The model under review builds one solid part; all positions refer to its coordinate system, in mm. Face numbers are marked on the shaded views. A direction names the side the tool comes from. Coordinates: 2 decimals unless noted, no trailing zeros. Write each loop counter-clockwise with the first axis right and the second up, starting at its lowest first coordinate (ties: lowest second). Pieces come first, ordered by that corner, then holes.
1) Add section A-A, the plane y = 0. State the section outline as (x, z) points.
2) Add section C-C, the plane x = -4. State the section outline as (y, z) points, then the cut area to 3 significant figures.
3) Add section B-B, the plane z = 5.75. State the section outline as (x, y) points, then the cut area to 3 significant figures.
4) Mouldability with a two-part tool opening along Z and no side actions: class the marked faces 3, 4 and 5 as released by +Z, released by -Z, zero draft, split by the parting line, or undercut.
5) Machinability: for the marked faces 1 and 2, which of the approach directions +Z, -Z, +X, -X, +Y, -Y give a long, thin tool a straight path to every point of the face, cutting with its end or side? Answer none if there is none.
6) For P1, Ø19.5, axis at x = -12.5, y = -21.65, coming from the +Z side; P2, Ø14.5, axis at x = -12.5, y = 21.65, coming from the +Z side; P3, Ø3, axis at x = -28.5, z = 10, coming from the +Y side; P4, Ø2, axis at y = 18.5, z = 9, coming from the -X side, all flat-tipped, find the tip position at first contact; note any pin that passes through.
7) Add section D-D, the plane y = -21.65. State the section outline as (x, z) points.
8) For line 1 (X direction, y = 6, z = 5.5); line 2 (Y direction, x = 0.5, z = 4.5); line 3 (Y direction, x = -12.5, z = 1.15), list the stretches that pass through material, from the lowest coordinate up.
from build123d import *

# Parameters (mm, degrees)
SKETCH_1_R     = 37.5
PAD_1_DEPTH    = 11
SKETCH_2_R     = 15
POCKET_2_DEPTH = 11.001
SKETCH_3_R     = 4.5
POCKET_3_DEPTH = 11.001
SKETCH_4_R     = 4.5
POCKET_4_DEPTH = 11.001
SKETCH_5_R     = 4.5
POCKET_5_DEPTH = 11.001
SKETCH_6_R     = 7.5
POCKET_6_DEPTH = 9
SKETCH_7_R     = 7.5
POCKET_7_DEPTH = 9
SKETCH_8_R     = 7.5
POCKET_8_DEPTH = 9


with BuildPart() as part:
    # Sketch_1 → Pad_1 (new body)
    with BuildSketch(Plane.XY):
        Circle(SKETCH_1_R)
    extrude(amount=PAD_1_DEPTH)

    # Sketch_2 (on Face3 of Pad_1) → Pocket_2 (cut, through all)
    with BuildSketch(Plane.XY.offset(11)):
        Circle(SKETCH_2_R)
    extrude(amount=-POCKET_2_DEPTH, mode=Mode.SUBTRACT)

    # Sketch_3 (on Face3 of Pocket_2) → Pocket_3 (cut, through all)
    with BuildSketch(Plane.XY.offset(11)):
        with Locations((25, 0)):
            Circle(SKETCH_3_R)
    extrude(amount=-POCKET_3_DEPTH, mode=Mode.SUBTRACT)

    # Sketch_4 (on Face3 of Pocket_3) → Pocket_4 (cut, through all)
    with BuildSketch(Plane.XY.offset(11)):
        with Locations((-12.5, 21.65)):
            Circle(SKETCH_4_R)
    extrude(amount=-POCKET_4_DEPTH, mode=Mode.SUBTRACT)

    # Sketch_5 (on Face3 of Pocket_4) → Pocket_5 (cut, through all)
    with BuildSketch(Plane.XY.offset(11)):
        with Locations((-12.5, -21.65)):
            Circle(SKETCH_5_R)
    extrude(amount=-POCKET_5_DEPTH, mode=Mode.SUBTRACT)

    # Sketch_6 (on Face3 of Pocket_5) → Pocket_6 (cut)
    with BuildSketch(Plane.XY.offset(11)):
        with Locations((25, 0)):
            Circle(SKETCH_6_R)
    extrude(amount=-POCKET_6_DEPTH, mode=Mode.SUBTRACT)

    # Sketch_7 (on Face3 of Pocket_6) → Pocket_7 (cut)
    with BuildSketch(Plane.XY.offset(11)):
        with Locations((-12.5, 21.65)):
            Circle(SKETCH_7_R)
    extrude(amount=-POCKET_7_DEPTH, mode=Mode.SUBTRACT)

    # Sketch_8 (on Face3 of Pocket_7) → Pocket_8 (cut)
    with BuildSketch(Plane.XY.offset(11)):
        with Locations((-12.5, -21.65)):
            Circle(SKETCH_8_R)
    extrude(amount=-POCKET_8_DEPTH, mode=Mode.SUBTRACT)


solid = part.part
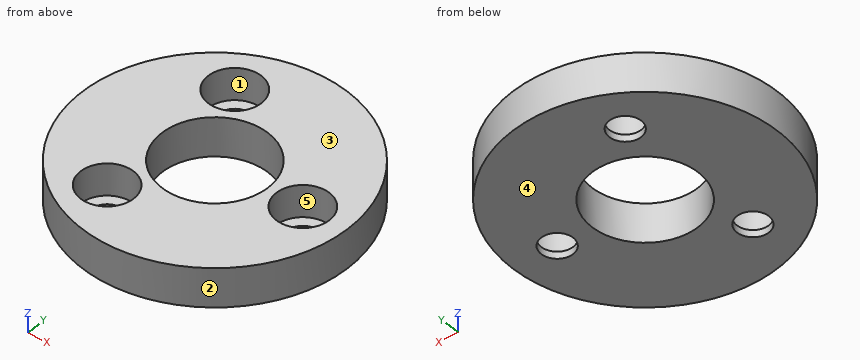
Geometry results:
1. outline: (-37.5, 0) - (-15, 0) - (-15, 11) - (-37.5, 11) - close; (15, 0) - (20.5, 0) - (20.5, 2) - (17.5, 2) - (17.5, 11) - (15, 11) - close; (29.5, 0) - (37.5, 0) - (37.5, 11) - (32.5, 11) - (32.5, 2) - (29.5, 2) - close
2. outline: (-37.29, 0) - (-14.46, 0) - (-14.46, 11) - (-37.29, 11) - close; (14.46, 0) - (37.29, 0) - (37.29, 11) - (14.46, 11) - close
2. area: 502 mm2
3. outline: circle Ø75 at (0, 0); hole circle Ø15 at (-12.5, -21.65); hole circle Ø15 at (-12.5, 21.65); hole circle Ø30 at (0, 0); hole circle Ø15 at (25, 0)
3. area: 3,180 mm2
4. face 3: released by +Z
4. face 4: released by -Z
4. face 5: zero draft
5. face 1: +Z
5. face 2: +Z, -Z
6. P1: stops at z = 11
6. P2: stops at z = 2
6. P3: stops at y = 26.02
6. P4: stops at x = -33.17
7. outline: (-30.62, 0) - (-17, 0) - (-17, 2) - (-20, 2) - (-20, 11) - (-30.62, 11) - close; (-8, 0) - (30.62, 0) - (30.62, 11) - (-5, 11) - (-5, 2) - (-8, 2) - close
8. line 1: x = -37.02 to -13.75, 13.75 to 20.5, 29.5 to 37.02
8. line 2: y = -37.5 to -14.99, 14.99 to 37.5
8. line 3: y = -35.36 to -26.15, -17.15 to -8.29, 8.29 to 17.15, 26.15 to 35.36
